```python
from build123d import *

# Parameters (mm, degrees)
SKETCH1_R           = 430
BOSS_EXTRUDE1_DEPTH = 12


with BuildPart() as part:
    # Sketch1 → Boss-Extrude1 (new body)
    with BuildSketch(Plane.XY):
        Circle(SKETCH1_R)
        with BuildLine():
            Line((413.001947093, 5.720930233), (409.96008459, 5.720930233))
            ThreePointArc((409.96008459, 5.720930233), (289.913780286, 289.913780286), (5.720930233, 409.96008459))
            Line((5.720930233, 409.96008459), (5.720930233, 413.001947093))
            Line((5.720930233, 413.001947093), (-5.720930233, 413.001947093))
            Line((-5.720930233, 413.001947093), (-5.720930233, 409.96008459))
            ThreePointArc((-5.720930233, 409.96008459), (-289.913780286, 289.913780286), (-409.96008459, 5.720930233))
            Line((-409.96008459, 5.720930233), (-413.001947093, 5.720930233))
            Line((-413.001947093, 5.720930233), (-413.001947093, -5.720930233))
            Line((-413.001947093, -5.720930233), (-409.96008459, -5.720930233))
            ThreePointArc((-409.96008459, -5.720930233), (-289.913780286, -289.913780286), (-5.720930233, -409.96008459))
            Line((-5.720930233, -409.96008459), (-5.720930233, -413.001947093))
            Line((-5.720930233, -413.001947093), (5.720930233, -413.001947093))
            Line((5.720930233, -413.001947093), (5.720930233, -409.96008459))
            ThreePointArc((5.720930233, -409.96008459), (289.913780286, -289.913780286), (409.96008459, -5.720930233))
            Line((409.96008459, -5.720930233), (413.001947093, -5.720930233))
            Line((413.001947093, -5.720930233), (413.001947093, 5.720930233))
        make_face(mode=Mode.SUBTRACT)
    extrude(amount=BOSS_EXTRUDE1_DEPTH)


solid = part.part
```
Here's how the part is built. I have some questions about the finished solid (model axes, mm). A direction names the side the tool comes from. Round coordinates to 2 decimals unless told otherwise and drop trailing zeros. Loops run counter-clockwise (first coordinate to the right, second up) from the corner with the lowest first, then second, coordinate; pieces in that order, holes last.
1. Will these pins go through, and if not, where does the flat tip stop? pin 1 (4 mm diameter, centred on x = -118.5, z = 2, fed in from +Y); pin 2 (3 mm diameter, centred on x = -209.5, z = 1.5, fed in from +Y); pin 3 (4 mm diameter, centred on y = -108.5, z = 4.5, fed in from +X).
Answers:
pin 1: stops at y = 413.92
pin 2: stops at y = 376.35
pin 3: stops at x = 416.6
2. For faces 1 (the face through (380, -157, 12)), 2 (the face through (286.766, -293.028, 5.916)), which set-ups out of +Z, -Z, +X, -X, +Y, -Y let a thin tool reach every point of the face, with its end or its side?
Answers:
face 1: +Z, +X, -X, +Y, -Y
face 2: +Z, -Z
3. Suppose I cut it at A-A, the plane x = -158.5. Please give me the cut outline in (y, z), and give its area (3 significant figures).
Answers:
outline: (-399.72, 0) - (-378.12, 0) - (-378.12, 12) - (-399.72, 12) - close; (378.12, 0) - (399.72, 0) - (399.72, 12) - (378.12, 12) - close
area: 518 mm2
4. Thinking about a two-plate mould opening in X: for faces 3 (the face through (380, -157, 0)), 4 (the face through (-341.23, -261.65, 5.92)), 5 (the face through (293.028, 286.766, 5.916)), which applies, released by +X, released by -X, zero draft, split by the parting line, or undercut?
Answers:
face 3: zero draft
face 4: split by the parting line
face 5: undercut
5. Suppose I cut it at C-C, the plane z = 5. Please give me the cut outline in (x, y), and give its area (3 significant figures).
Answers:
outline: circle Ø860 at (0, 0); hole (-413, -5.72) - (-409.96, -5.72) arc R410 ccw to (-5.72, -409.96) - (-5.72, -413) - (5.72, -413) - (5.72, -409.96) arc R410 ccw to (409.96, -5.72) - (413, -5.72) - (413, 5.72) - (409.96, 5.72) arc R410 ccw to (5.72, 409.96) - (5.72, 413) - (-5.72, 413) - (-5.72, 409.96) arc R410 ccw to (-409.96, 5.72) - (-413, 5.72) - close
area: 52,600 mm2
6. If I drill on probe 1 along X at (y, z) = (66, 6); probe 2 along X at (y, z) = (11, 3.25); probe 3 along Y at (x, z) = (308, 11), over which ranges is the centre line in solid material (lowest first)?
Answers:
probe 1: x = -424.9 to -404.65, 404.65 to 424.9
probe 2: x = -429.86 to -409.85, 409.85 to 429.86
probe 3: y = -300.06 to -270.62, 270.62 to 300.06
7. Suppose I cut it at B-B, the plane y = -320. Please give me the cut outline in (x, z).
Answers:
outline: (-287.23, 0) - (-256.32, 0) - (-256.32, 12) - (-287.23, 12) - close; (256.32, 0) - (287.23, 0) - (287.23, 12) - (256.32, 12) - close
